Design review of the part shown in the three views and the two pictorial views. Dimensions are in mm from the part's minimum x, y and z. A direction names the side the tool comes from. Give positions to 0.01 mm unless a question says otherwise; leave off trailing zeros. Write each loop counter-clockwise with the first axis right and the second up, starting at its lowest first coordinate (ties: lowest second). Pieces come first, ordered by that corner, then holes. Notation, with made-up numbers: M -33.5,59.5 L 8.5,59.5 A12 cw 8.5,74.5 Z; hole C -2.75,24 d5. An arc over 180 degrees is marked long. Write item = value, one per line.
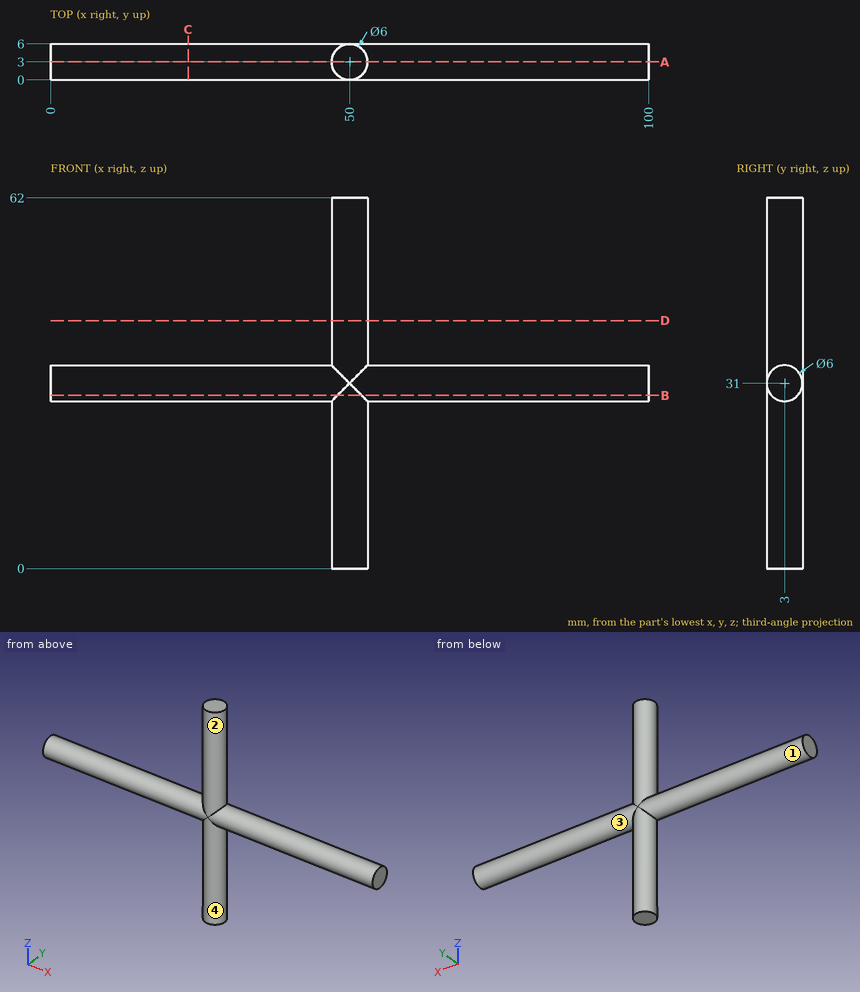
1. We need section A-A, the plane y = 3. Write out the cut boundary in (x, z).
Responses:
outline = M 0,28 L 47,28 L 47,0 L 53,0 L 53,28 L 100,28 L 100,34 L 53,34 L 53,62 L 47,62 L 47,34 L 0,34 Z
2. We need section C-C, the plane x = 23. Write out the cut boundary in (y, z).
Responses:
outline = C 3,31 d6
3. For line 1 along Z through (x, y) = (68, 3.15); line 2 along X through (y, z) = (3.2, 55); line 3 along X through (y, z) = (3.75, 12.5), list the stretches that pass through material, from the lowest coordinate up. Write a range as from..to.
Responses:
line_1 = 28..34
line_2 = 47.01..52.99
line_3 = 47.1..52.9
4. Machinability: for the marked faces 1, 2, 3 and 4, which of the approach directions +Z, -Z, +X, -X, +Y, -Y give a long, thin tool a straight path to every point of the face, cutting with its end or side? Answer none if there is none.
Responses:
face_1 = -X
face_2 = +Z
face_3 = +X
face_4 = -Z
5. Insertion check: P1, Ø1, axis at x = 53.5, y = 1.5, coming from the -Z side; P2, Ø1, axis at y = 2.5, z = 21.5, coming from the +X side; P3, Ø3, axis at x = 47.5, z = 17, coming from the +Y side. Each pin has a flat end and moves straight along its axis. Give the tip position at first contact, or say it passes through.
Responses:
P1 = 28.17
P2 = 53
P3 = 5.83
6. We need section B-B, the plane z = 29. Write out the cut boundary in (x, y).
Responses:
outline = M 0,0.76 L 48,0.76 A3 ccw 52,0.76 L 100,0.76 L 100,5.24 L 52,5.24 A3 ccw 48,5.24 L 0,5.24 Z
7. We need section D-D, the plane z = 41.5. Write out the cut boundary in (x, y).
Responses:
outline = C 50,3 d6
